Verification items for the finished model (mm, model axes). A direction names the side the tool comes from. Give positions to 0.01 mm unless a question says otherwise; leave off trailing zeros. Write each loop counter-clockwise with the first axis right and the second up, starting at its lowest first coordinate (ties: lowest second). Pieces come first, ordered by that corner, then holes. Notation, with made-up numbers: (72.25, 46) -> (108.25, 46) arc R15 ccw to (108.25, 66) -> close; hole circle Ø10 at (-29, -21.5). An arc over 180 degrees is marked (long way). Use one line per item in the form item = value. Start each with the question number.
(1) Release check for a two-part mould opening along Y. For faces 4 (the face through (4.194, 0.047, -0.212)), 5 (the face through (-1.11, -0.27, -1.22)), 6 (the face through (9.973, 0, 0)), 7 (the face through (-2, 3, 0)) record: pulls with the +Y half, pulls with the -Y half, needs draft (parallel to the pull), parting line crosses it, or undercut.
(2) Section check B-B, the plane y = 3.75. Record the cut outline in (x, z).
(3) Depth check by flat-ended pin: pin 1 Ø1 at (x, y) = (1.5, -2.5) entering from +Z; pin 2 Ø4 at (x, z) = (1.5, -2.5) entering from -Y; pin 3 Ø1.3 at (x, z) = (-1.5, 0.5) entering from +Y. Enter the tip coordinate at first touch or a pass-through.
(4) Scan lines: L1, parallel to Z at x = -1, y = 0; L2, parallel to X at y = -0.25, z = 3.25. Record each from-to range of solid material in increasing order.
(5) Set-up check for faces 1 (the face through (9, 0, -3)), 2 (the face through (-2, -3, 0)), 3 (the face through (8.03, -2.44, -0.54)): record each of +Z, -Z, +X, -X, +Y, -Y from which the full face is reachable in a straight line by a thin tool's end or side.
(6) Section check A-A, the plane z = 3.75. Record the cut outline in (x, y).
from build123d import *

# Parameters (mm, degrees)
F2_W     = 4
F2_H     = 10
F3_DEPTH = 2.5
F5_D     = 2.5
F5_DEPTH = 9.5
F5_TIP   = 0.7510757738
F6_W     = 0.9
F6_H     = 2
F8_SIZE  = 0.3


with BuildPart() as f1:
    # F0 (on Front) → F1 (revolve)
    with BuildSketch(Plane.XZ):
        Polygon((-5.9266670129, 2.1), (-5.9266670129, 0), (9.9733329871, 0), (9.9733329871, 3), (0.3733329871, 3), (0.3733329871, 4), (-3.1266670129, 4), (-3.1266670129, 2.1), align=None)
    revolve(axis=Axis((2.0233329871, 0, 0), (-1, 0, 0)))

    # F2 (on face) → F3 (cut)
    with BuildSketch(Plane(origin=(-3.1266670129, 0, 0), x_dir=(0, -1, 0), z_dir=(-1, 0, 0))):
        with Locations((5, 0)):
            Rectangle(F2_W, F2_H)
        with Locations((-5, 0)):
            Rectangle(F2_W, F2_H)
    extrude(amount=-F3_DEPTH, mode=Mode.SUBTRACT)

    # F5
    with Locations(Plane(origin=(-5.9266670129, 0, 0), x_dir=(0, -1, 0), z_dir=(-1, 0, 0))):
        with Locations((0, 0)):
            Hole(F5_D / 2, depth=F5_DEPTH)
            with Locations((0, 0, -(F5_DEPTH + F5_TIP / 2))):  # 118° drill point
                Cone(0, F5_D / 2, F5_TIP, mode=Mode.SUBTRACT)

    # F6 (on Front) → F7 (revolve, cut)
    with BuildSketch(Plane.XZ):
        with Locations((8.0233329871, 3.5)):
            Rectangle(F6_W, F6_H)
    revolve(axis=Axis((2.0233329871, 0, 0), (-1, 0, 0)), mode=Mode.SUBTRACT)

    # F8
    f8_edges = [f1.edges().sort_by_distance(p)[0] for p in [
        (9.973333, 0, -3),
        (-5.926667, 0, -2.1),
    ]]
    chamfer(f8_edges, length=F8_SIZE)


solid = f1.part
Completed:
q1.face_4 = undercut
q1.face_5 = undercut
q1.face_6 = needs draft
q1.face_7 = pulls with the +Y half
q2.outline = (-0.63, -1.39) -> (0.37, -1.39) -> (0.37, 1.39) -> (-0.63, 1.39) -> close
q3.pin_1 = 2.24
q3.pin_2 = -3.91
q3.pin_3 = 3
q4.L1 = -4 to -1.25, 1.25 to 4
q4.L2 = -3.13 to 0.37
q5.face_1 = +X
q5.face_2 = +Z, -Z, -X, -Y
q5.face_3 = none
q6.outline = (-3.13, -1.39) -> (0.37, -1.39) -> (0.37, 1.39) -> (-3.13, 1.39) -> close
